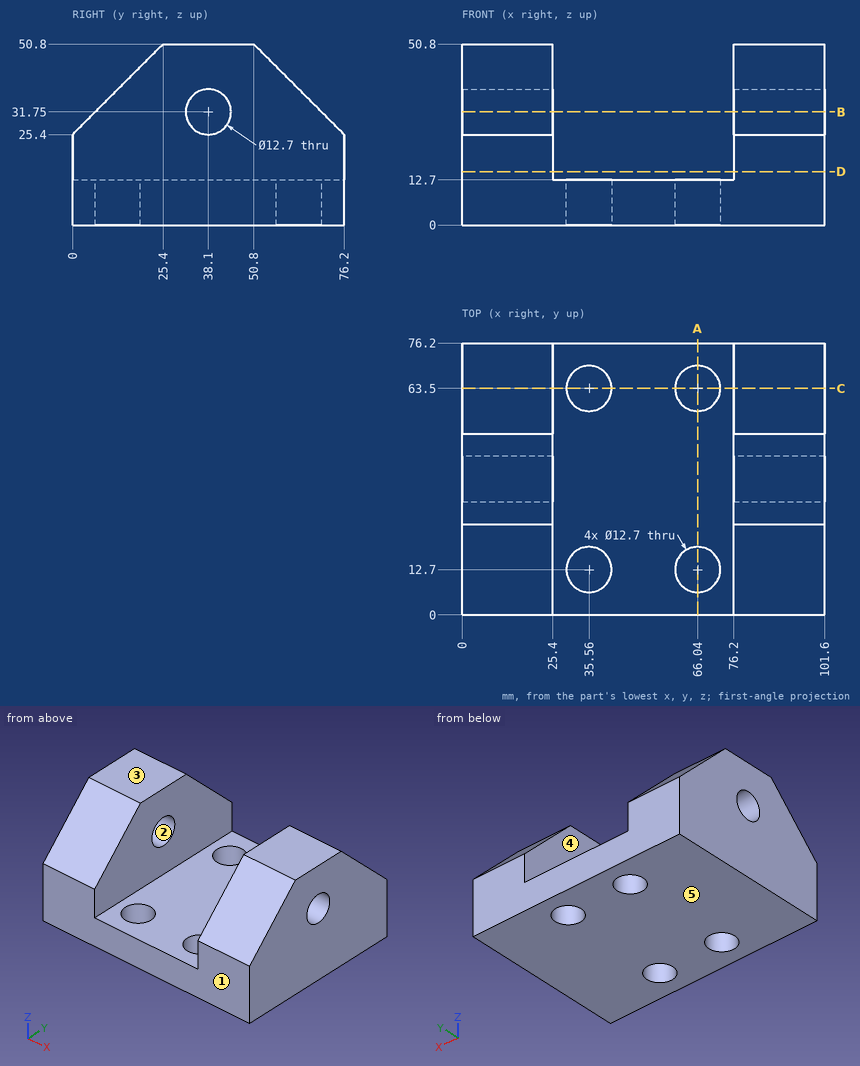
Here's the drawing with two shaded views (mm, measured from the low corner). I have some questions. A direction names the side the tool comes from. Give positions to 0.01 mm unless a question says otherwise; leave off trailing zeros. Order: outer loops, then holes, each group sorted by start corner. A loop starts at its lowest first (then second) coordinate and runs counter-clockwise, first axis right, second up.
Q1. We'd pull the mould along Z, two halves only. Please class the marked faces 1, 2 and 3: +Z half, -Z half, draft (parallel to the pull), parting line (faces both ways), or undercut.
Q2. I'm going to push flat-ended pins straight in: P1, Ø6, axis at x = 14.5, y = 58, coming from the -Z side; P2, Ø3, axis at x = 45, y = 10.5, coming from the +Z side. Where does each tip first touch, or does it pass through?
Q3. Suppose I cut it at C-C, the plane y = 63.5. Write out the boundary of the cut face in (x, z).
Q4. For the marked faces 4 and 5, which set-ups out of +Z, -Z, +X, -X, +Y, -Y let a thin tool reach every point of the face, with its end or its side?
Q5. If I drill on line 1 along Y through (x, z) = (66.04, 5.5); line 2 along Z through (x, y) = (94, 38); line 3 along X through (y, z) = (18, 24), over which ranges is the centre line in solid material (lowest first)?
Q6. Suppose I cut it at D-D, the plane z = 15. Write out the boundary of the cut face in (x, y), and give its area (3 significant figures).
Q7. Suppose I cut it at B-B, the plane z = 31.75. Write out the boundary of the cut face in (x, y).
Q8. Suppose I cut it at A-A, the plane x = 66.04. Write out the boundary of the cut face in (y, z).
Solution:
1. face 1: draft
1. face 2: undercut
1. face 3: +Z half
2. P1: stops at z = 0
2. P2: stops at z = 12.7
3. outline: (0, 0) - (29.21, 0) - (29.21, 12.7) - (25.4, 12.7) - (25.4, 38.1) - (0, 38.1) - close; (41.91, 0) - (59.69, 0) - (59.69, 12.7) - (41.91, 12.7) - close; (72.39, 0) - (101.6, 0) - (101.6, 38.1) - (76.2, 38.1) - (76.2, 12.7) - (72.39, 12.7) - close
4. face 4: +Z, +Y, -Y
4. face 5: -Z, +X, -X, +Y, -Y
5. line 1: y = 0 to 6.35, 19.05 to 57.15, 69.85 to 76.2
5. line 2: z = 0 to 25.4, 38.1 to 50.8
5. line 3: x = 0 to 25.4, 76.2 to 101.6
6. outline: (0, 0) - (25.4, 0) - (25.4, 76.2) - (0, 76.2) - close; (76.2, 0) - (101.6, 0) - (101.6, 76.2) - (76.2, 76.2) - close
6. area: 3,870 mm2
7. outline: (0, 6.35) - (25.4, 6.35) - (25.4, 31.75) - (0, 31.75) - close; (0, 44.45) - (25.4, 44.45) - (25.4, 69.85) - (0, 69.85) - close; (76.2, 6.35) - (101.6, 6.35) - (101.6, 31.75) - (76.2, 31.75) - close; (76.2, 44.45) - (101.6, 44.45) - (101.6, 69.85) - (76.2, 69.85) - close
8. outline: (0, 0) - (6.35, 0) - (6.35, 12.7) - (0, 12.7) - close; (19.05, 0) - (57.15, 0) - (57.15, 12.7) - (19.05, 12.7) - close; (69.85, 0) - (76.2, 0) - (76.2, 12.7) - (69.85, 12.7) - close
